from build123d import *

# Parameters (mm, degrees)
C_CHANNEL_120_X_12_1_DEPTH = 600


with BuildPart() as part:
    # Sketch11 → C channel 120 X 12(1) (new body)
    with BuildSketch(Plane(origin=(0, 0, 0), x_dir=(0, -1, 0), z_dir=(-1, 0, 0))):
        with BuildLine():
            Line((65, 125), (0, 125))
            Line((0, 125), (0, 0))
            Line((0, 0), (65, 0))
            Line((65, 0), (65, 5.845330836))
            ThreePointArc((65, 5.845330836), (63.844151715, 8.856418565), (60.970378085, 10.320679365))
            Line((60.970378085, 10.320679365), (13.463772294, 15.313824837))
            ThreePointArc((13.463772294, 15.313824837), (8.354841396, 17.916955149), (6.3, 23.27))
            Line((6.3, 23.27), (6.3, 106.74))
            ThreePointArc((6.3, 106.74), (8.354841396, 112.093044851), (13.463772294, 114.696175163))
            Line((13.463772294, 114.696175163), (60.970378085, 119.689320635))
            ThreePointArc((60.970378085, 119.689320635), (63.844151715, 121.153581435), (65, 124.164669164))
            Line((65, 124.164669164), (65, 125))
        make_face()
    extrude(amount=C_CHANNEL_120_X_12_1_DEPTH)


solid = part.part
Geometry check sheet. Reference: the model listing, model coordinates, mm. A direction names the side the tool comes from. Coordinates: 2 decimals unless noted, no trailing zeros. Order: outer loops, then holes, each group sorted by start corner. A loop starts at its lowest first (then second) coordinate and runs counter-clockwise, first axis right, second up. Notation, with made-up numbers: (18, -22.5) - (33, -22.5) arc R27 ccw to (33, 12.5) - close; hole circle Ø11 at (54.5, 73.25). An arc over 180 degrees is marked (long way). Answer in a Markdown table with one row per item. Add a question column.
1) Material ranges on line 1 along Z through (x, y) = (-158, -61.5); line 2 along Y through (x, z) = (-91, 87); line 3 along Z through (x, y) = (-572, -26), recorded low to high. Write a range as [from, to].
2) Gauge pin test, flat ends, axial feed: P1, Ø25, axis at x = -246.5, z = 80.5, coming from the -Y side; P2, Ø5, axis at y = -10.5, z = 67.5, coming from the -X side. Record the tip position at first contact, or that the pin passes through.
3) Cross-section at B-B, the plane x = -223. Record the cut outline in (y, z).
4) Release check for a two-part mould opening along Z. For faces 3 (the flat face through (-295.8, -36.885, 117.158)), 4 (the flat face through (-296, -32, 0)), 5 (the flat face through (-600, -6, 54)) record: +Z half, -Z half, draft (parallel to the pull), parting line (faces both ways), or undercut.
5) Cross-section at D-D, the plane y = -51.5. Record the cut outline in (x, z), then the cut area to 3 significant figures.
6) Cross-section at C-C, the plane z = 66. Record the cut outline in (x, y).
7) Cross-section at A-A, the plane y = -28.5. Record the cut outline in (x, z).
8) Set-up check for faces 1 (the flat face through (0, -6, 54)), 2 (the flat face through (-296, -6.3, 64)): record each of +Z, -Z, +X, -X, +Y, -Y from which the full face is reachable in a straight line by a thin tool's end or side.
Check result:
| question | item | result |
|---|---|---|
| 1 | line 1 | z = [0, 10.23], [119.78, 125] |
| 1 | line 2 | y = [-6.3, 0] |
| 1 | line 3 | z = [0, 14], [116.01, 125] |
| 2 | P1 | stops at y = -6.3 |
| 2 | P2 | passes through |
| 3 | outline | (-65, 0) - (0, 0) - (0, 125) - (-65, 125) - (-65, 124.16) arc R4.5 ccw to (-60.97, 119.69) - (-13.46, 114.7) arc R8 cw to (-6.3, 106.74) - (-6.3, 23.27) arc R8 cw to (-13.46, 15.31) - (-60.97, 10.32) arc R4.5 ccw to (-65, 5.85) - close |
| 4 | face 3 | undercut |
| 4 | face 4 | -Z half |
| 4 | face 5 | draft |
| 5 | outline | (-600, 0) - (0, 0) - (0, 11.32) - (-600, 11.32) - close; (-600, 118.69) - (0, 118.69) - (0, 125) - (-600, 125) - close |
| 5 | area | 10,600 mm² |
| 6 | outline | (-600, -6.3) - (0, -6.3) - (0, 0) - (-600, 0) - close |
| 7 | outline | (-600, 0) - (0, 0) - (0, 13.73) - (-600, 13.73) - close; (-600, 116.28) - (0, 116.28) - (0, 125) - (-600, 125) - close |
| 8 | face 1 | +Z, -Z, +X, +Y, -Y |
| 8 | face 2 | +X, -X, -Y |
